Autodesk Inventor part; units mm, degrees
ref_plane "YZ Plane" through (0, 0, 0) normal (1, 0, 0) x (0, 1, 0)
ref_plane "XZ Plane" through (0, 0, 0) normal (0, 1, 0) x (-1, 0, 0)
ref_plane "XY Plane" through (0, 0, 0) normal (0, 0, 1) x (1, 0, 0)
sketch "Sketch1" plane through (0, 0, 0) normal (0, 0, 1) x (1, 0, 0)
  line L0 (0, 0) -> (12, 0) construction
  line L1 (12, 0) -> (12, 30)
  line L2 (12, 30) -> (0, 30) construction
  line L3 (0, 30) -> (0, 0)
  arc A0 (12, 30) -> (0, 30) centre (6, 30) ccw
  arc A1 (0, 0) -> (12, 0) centre (6, 0) ccw
  circle A2 centre (6, 30) radius 1.5
  circle A3 centre (6, 0) radius 1.5
  dimension "d0" = 12
  dimension "d1" = 30
  dimension "d2" = 3
  dimension "d3" = 3
extrude "Extrusion1" add sketch "Sketch1" along normal blind 4
properties part number "z axis arm1"
Geometry: final body of the model. Coordinates: model frame, mm. Round coordinates to 2 decimals unless told otherwise and drop trailing zeros. Order: outer loops, then holes, each group sorted by start corner. A loop starts at its lowest first (then second) coordinate and runs counter-clockwise, first axis right, second up. Notation, with made-up numbers: (42, 15.5) -> (99, 15.5) arc R21 ccw to (99, 23.5) -> close; hole circle Ø9 at (2.5, 60). An arc over 180 degrees is marked (long way). Use CSV: the item, a comma, the result in double quotes. Start each with the question number.
1) Draft query along Y for faces 1 (the face through (6, 36, 2)), 2 (the face through (4.8, 0.9, 2)), 3 (the face through (6, 15, 0)). Return one class per face: +Y half, -Y half, draft (parallel to the pull), parting line (faces both ways), or undercut.
2) Material intervals for line 1 along Y through (x, z) = (6, 1.1); line 2 along Y through (x, z) = (5.5, 2.2); line 3 along Y through (x, z) = (11.25, 2.9), sorted ascending. Write a range as from..to.
3) First-contact query: pin 1 Ø1 at (y, z) = (26.5, 2.5) entering from -X; pin 2 Ø2 at (x, z) = (2, 3.5) entering from -Y; pin 3 Ø1.5 at (x, z) = (5, 0.5) entering from +Y. Flat tips, straight axial feed; report the tip coordinate or a pass-through.
4) Section A-A (x = 6). Return the cut outline in (y, z), and give its area (3 significant figures).
5) Section B-B (z = 1.25). Return the cut outline in (x, y).
6) Section C-C (x = 9). Return the cut outline in (y, z).
Returned:
1,face 1,"+Y half"
1,face 2,"undercut"
1,face 3,"draft"
2,line 1,"y = -6..-1.5, 1.5..28.5, 31.5..36"
2,line 2,"y = -5.98..-1.41, 1.41..28.59, 31.41..35.98"
2,line 3,"y = -2.9..32.9"
3,pin 1,"stops at x = 0"
3,pin 2,"stops at y = -5.2"
3,pin 3,"stops at y = 35.99"
4,outline,"(-6, 0) -> (-1.5, 0) -> (-1.5, 4) -> (-6, 4) -> close; (1.5, 0) -> (28.5, 0) -> (28.5, 4) -> (1.5, 4) -> close; (31.5, 0) -> (36, 0) -> (36, 4) -> (31.5, 4) -> close"
4,area,"144 mm²"
5,outline,"(0, 0) arc R6 ccw to (12, 0) -> (12, 30) arc R6 ccw to (0, 30) -> close; hole circle Ø3 at (6, 0); hole circle Ø3 at (6, 30)"
6,outline,"(-5.2, 0) -> (35.2, 0) -> (35.2, 4) -> (-5.2, 4) -> close"
